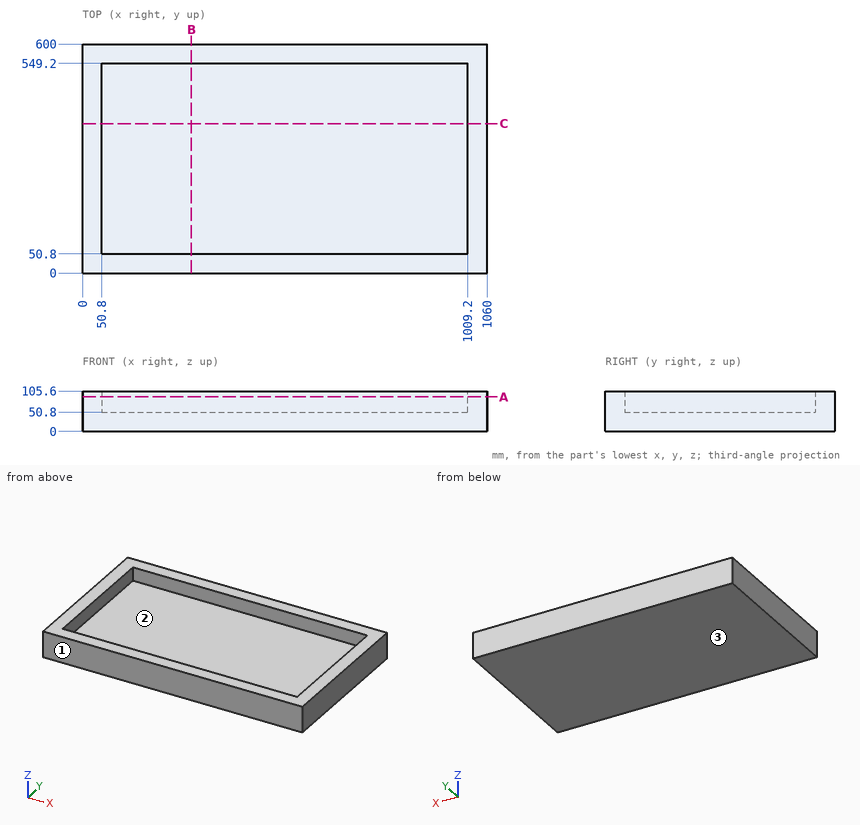
Job drawing, mm, ordinate dimensions from the low corner. One solid piece. Round coordinates to 2 decimals unless told otherwise and drop trailing zeros. Loops run counter-clockwise (first coordinate to the right, second up) from the corner with the lowest first, then second, coordinate; pieces in that order, holes last.
Item 1: Mould opens along Y. For the marked faces 1, 2 and 3 say: +Y half, -Y half, draft (parallel to the pull), parting line (faces both ways), or undercut.
Item 2: Cut at B-B, the plane x = 285. Give the cut face in (y, z).
Item 3: Cut at C-C, the plane y = 391.5. Give the cut face in (x, z).
Item 4: Cut at A-A, the plane z = 90.5. Give the cut face in (x, y).
Item 5: Drop a flat-ended pin along its axis: P1, Ø4, axis at x = 326.5, y = 504, coming from the +Z side. Give the stop position or say it passes through.
Item 6: Drill centre lines: line 1 (Y direction, x = 130, z = 80); line 2 (X direction, y = 510.5, z = 86); line 3 (Z direction, x = 244.5, y = 222). Where is each one in solid material? Low to high.
A:
1. face 1: -Y half
1. face 2: undercut
1. face 3: draft
2. outline: (0, 0) - (600, 0) - (600, 105.6) - (549.2, 105.6) - (549.2, 50.8) - (50.8, 50.8) - (50.8, 105.6) - (0, 105.6) - close
3. outline: (0, 0) - (1060, 0) - (1060, 105.6) - (1009.2, 105.6) - (1009.2, 50.8) - (50.8, 50.8) - (50.8, 105.6) - (0, 105.6) - close
4. outline: (0, 0) - (1060, 0) - (1060, 600) - (0, 600) - close; hole (50.8, 50.8) - (1009.2, 50.8) - (1009.2, 549.2) - (50.8, 549.2) - close
5. P1: stops at z = 50.8
6. line 1: y = 0 to 50.8, 549.2 to 600
6. line 2: x = 0 to 50.8, 1009.2 to 1060
6. line 3: z = 0 to 50.8
